Check sheet for the modelled part. Datum: model origin and axes. Units: mm. A direction names the side the tool comes from. Round coordinates to 2 decimals unless told otherwise and drop trailing zeros. Loops run counter-clockwise (first coordinate to the right, second up) from the corner with the lowest first, then second, coordinate; pieces in that order, holes last. Notation, with made-up numbers: (88.25, 45.25) - (134.25, 45.25) arc R24 ccw to (134.25, 77.25) - close; hole circle Ø10 at (-2, 75). An arc over 180 degrees is marked (long way). Put each result on its own line as item: value. Start each with the question number.
Item 1: Draft check along Z on faces 3 (the flat face through (-0.3, -50.8, -8.4)), 4 (the flat face through (0, -25.4, 0)), 5 (the flat face through (0, -13, -41.319)). Enter one of: pulls with the +Z half, pulls with the -Z half, needs draft (parallel to the pull), parting line crosses it, or undercut.
Item 2: Tool access check on faces 1 (the cylindrical face through (-1.755, -37.922, -7.905)), 2 (the flat face through (-43.947, -13, -2)). Record the directions out of +Z, -Z, +X, -X, +Y, -Y that give a thin tool (end or side, any length) a straight path to the whole face; none if there is none.
Item 3: Section check A-A, the plane x = 0. Record the cut outline in (y, z).
Item 4: Section check B-B, the plane z = 0. Record the cut outline in (x, y), and give its area (3 significant figures).
Item 5: Gauge pin test, flat ends, axial feed: pin 1 Ø14.5 at (x, z) = (0, 0) entering from -Y; pin 2 Ø10 at (x, y) = (20, -40.5) entering from +Z; pin 3 Ø5 at (x, y) = (-17, -34.5) entering from -Z. Record the tip position at first contact, or that the pin passes through.
Item 6: Section check C-C, the plane z = -13.5. Record the cut outline in (x, y).
Item 7: Section check D-D, the plane x = -12. Record the cut outline in (y, z), and give its area (3 significant figures).
Item 8: Material ranges on line 1 along X through (y, z) = (-31.5, 0); line 2 along Y through (x, z) = (5, -1.5), recorded low to high.
from build123d import *

# Parameters (mm, degrees)
F0_R     = 19.4628925801
F0_R_2   = 14.0890060642
F0_R_3   = 8.0974467075
F1_DEPTH = 50.8
F2_W     = 88.7702181935
F2_H     = 79.4259868562
F3_DEPTH = 25.4


with BuildPart() as f1:
    # F0 (on Front) → F1 (new body)
    with BuildSketch(Plane.XZ):
        Circle(F0_R)
        Circle(F0_R_2, mode=Mode.SUBTRACT)
        Circle(F0_R_2)
        Circle(F0_R_3, mode=Mode.SUBTRACT)
    extrude(amount=F1_DEPTH)

    # F2 (on Front) → F3 (join)
    with BuildSketch(Plane.XZ):
        with Locations((0.4380121827, -1.6060378402)):
            Rectangle(F2_W, F2_H)
    extrude(amount=F3_DEPTH)


solid = f1.part
Check result:
1. face 3: needs draft
1. face 4: undercut
1. face 5: pulls with the -Z half
2. face 1: -Y
2. face 2: +Z, -Z, -X, +Y, -Y
3. outline: (-50.8, -19.46) - (-25.4, -19.46) - (-25.4, -41.32) - (0, -41.32) - (0, 38.11) - (-25.4, 38.11) - (-25.4, 19.46) - (-50.8, 19.46) - (-50.8, 8.1) - (-25.4, 8.1) - (-25.4, -8.1) - (-50.8, -8.1) - close
4. outline: (-43.95, -25.4) - (-19.46, -25.4) - (-19.46, -50.8) - (-8.1, -50.8) - (-8.1, -25.4) - (8.1, -25.4) - (8.1, -50.8) - (19.46, -50.8) - (19.46, -25.4) - (44.82, -25.4) - (44.82, 0) - (-43.95, 0) - close
4. area: 2,830 mm²
5. pin 1: y = -25.4
5. pin 2: z = 12.4
5. pin 3: z = -12.98
6. outline: (-43.95, -25.4) - (-14.02, -25.4) - (-14.02, -50.8) - (14.02, -50.8) - (14.02, -25.4) - (44.82, -25.4) - (44.82, 0) - (-43.95, 0) - close
7. outline: (-50.8, -15.32) - (-25.4, -15.32) - (-25.4, -41.32) - (0, -41.32) - (0, 38.11) - (-25.4, 38.11) - (-25.4, 15.32) - (-50.8, 15.32) - close
7. area: 2,800 mm²
8. line 1: -19.46 to -8.1, 8.1 to 19.46
8. line 2: -25.4 to 0
